Work out the finished part from the listing and answer in its coordinate system (mm). A direction names the side the tool comes from. Coordinates: 2 decimals unless noted, no trailing zeros. Loops run counter-clockwise (first coordinate to the right, second up) from the corner with the lowest first, then second, coordinate; pieces in that order, holes last. Notation, with made-up numbers: (58, -6.75) - (98, -6.75) arc R21 ccw to (98, 6.25) - close; hole circle Ø9 at (31, 38.25). An arc over 180 degrees is marked (long way). Write each question's results on one line, items separated by ' | '. Start each with the question number.
1. Determine the mould class of faces 1 (the flat face through (-5, 33.5, 6)), 2 (the flat face through (0, 32, -7.874)), 3 (the conical face through (-0.36, 33.36, 8.63)) for opening direction X: released by +X, released by -X, zero draft, split by the parting line, or undercut.
2. A cutting plane is placed at C-C on y = 29.25. Determine the outline of the cut face in (x, z).
3. Which of the six approach directions +Z, -Z, +X, -X, +Y, -Y give full straight-line access (tool end or side, diameter ignored) to faces 4 (the cylindrical face through (0, 30, -8)), 5 (the flat face through (-1, 30, -8.646)), 6 (the flat face through (7.416, 2.508, 4.325)), 7 (the flat face through (0, 3, -8.585)), 8 (the flat face through (-7.154, 3.6, 4.78))?
4. A cutting plane is placed at A-A on x = 0. Determine the outline of the cut face in (y, z).
5. A cutting plane is placed at D-D on y = 5.5. Determine the outline of the cut face in (x, z), then the cut area to 3 significant figures.
6. Each of these flat-tipped pins is pushed along its axis until it touches: P1, Ø2.5, axis at x = -0.5, y = 1.5, coming from the -Z side; P2, Ø2, axis at x = 3, z = 5, coming from the -Y side; P3, Ø1, axis at y = 4, z = 4.5, coming from the -X side; P4, Ø5, axis at y = 7, z = 6.5, coming from the +X side. Where does it stop, or does it pass through?
7. Find the intervals of material crossed by line 1 along X through (y, z) = (20.5, 0); line 2 along Y through (x, z) = (0, -8.1), in increasing order. Write a range as [from, to].
8. A cutting plane is placed at B-B on z = 0. Determine the outline of the cut face in (x, y), then the cut area to 3 significant figures.
from build123d import *

# Parameters (mm, degrees)
ESQUISSE1_R                  = 9
ESQUISSE1_R_2                = 7
BOSS_EXTRU_1_DEPTH           = 33.5
ENL_V_MAT_EXTRU_1_DEPTH      = 5
ESQUISSE3_R                  = 1
ENL_V_MAT_EXTRU_2_DEPTH      = 1.65725
ENL_V_START                  = -3
ENL_V_MAT_EXTRU_6_DEPTH      = 3
ENL_V_START_2                = -5.5
ENL_V_MAT_EXTRU_3_DEPTH      = 5.5
ENL_V_MAT_EXTRU_4_REACH      = 40.918
ENL_V_MAT_EXTRU_4_END_RADIUS = 7
ESQUISSE5_R                  = 0.75
CHANFREIN2_SIZE              = 0.5


with BuildPart() as part:
    # Esquisse1 → Boss.-Extru.1 (new body)
    with BuildSketch(Plane(origin=(0, 0, 0), x_dir=(1, 0, 0), z_dir=(0, 1, 0))):
        with Locations(Location((0, 0, 0), (0, 0, 270))):
            Circle(ESQUISSE1_R)
        with Locations(Location((0, 0, 0), (0, 0, 270))):
            Circle(ESQUISSE1_R_2, mode=Mode.SUBTRACT)
    extrude(amount=BOSS_EXTRU_1_DEPTH)

    # Esquisse2 → Enlèv. mat.-Extru.1 (cut)
    with BuildSketch(Plane.XZ):
        with BuildLine():
            Line((2.7, -8.585452813), (-2.7, -8.585452813))
            ThreePointArc((-2.7, -8.585452813), (0, -9), (2.7, -8.585452813))
        make_face()
        with BuildLine():
            Line((-8.785220239, 1.954457816), (-6.085220239, 6.630994997))
            ThreePointArc((-6.085220239, 6.630994997), (-7.794228634, 4.5), (-8.785220239, 1.954457816))
        make_face()
        with BuildLine():
            Line((6.085220239, 6.630994997), (8.785220239, 1.954457816))
            ThreePointArc((8.785220239, 1.954457816), (7.794228634, 4.5), (6.085220239, 6.630994997))
        make_face()
    extrude(amount=-ENL_V_MAT_EXTRU_1_DEPTH, mode=Mode.SUBTRACT)

    # Esquisse3 → Enlèv. mat.-Extru.2 (cut)
    with BuildSketch(Plane(origin=(-7.435220239, 0, 4.292726406), x_dir=(-0.49999999999999967, 0, -0.8660254037844389), z_dir=(0.8660254037844389, 0, -0.49999999999999967))):
        with Locations(Location((0, 2.5, 0), (0, 0, 180))):
            Circle(ESQUISSE3_R)
    extrude(amount=ENL_V_MAT_EXTRU_2_DEPTH, mode=Mode.SUBTRACT)

    # Esquisse8 → Enlèv. mat.-Extru.6 (cut)
    with BuildSketch(Plane(origin=(0, 33.5, 0), x_dir=(1, 0, 0), z_dir=(0, 1, 0)).offset(ENL_V_START)):
        with BuildLine():
            Line((-1.5, 8.874119675), (-1.5, 7.874119675))
            Line((-1.5, 7.874119675), (1.5, 7.874119675))
            Line((1.5, 7.874119675), (1.5, 8.874119675))
            ThreePointArc((1.5, 8.874119675), (0, 9), (-1.5, 8.874119675))
        make_face()
    extrude(amount=ENL_V_MAT_EXTRU_6_DEPTH, mode=Mode.SUBTRACT)

    # Esquisse4 → Enlèv. mat.-Extru.3 (cut)
    with BuildSketch(Plane(origin=(0, 33.5, 0), x_dir=(1, 0, 0), z_dir=(0, 1, 0)).offset(ENL_V_START_2)):
        with BuildLine():
            Line((2.5, 8.645808233), (-2.5, 8.645808233))
            ThreePointArc((-2.5, 8.645808233), (0, 9), (2.5, 8.645808233))
        make_face()
    extrude(amount=ENL_V_MAT_EXTRU_3_DEPTH, mode=Mode.SUBTRACT)

    # Enlèv. mat.-Extru.4: up to this cylinder (the profile starts outside it)
    enl_v_mat_extru_4_end = Plane(origin=(0, 29.25, 0), z_dir=(0, -1, 0)) * Cylinder(ENL_V_MAT_EXTRU_4_END_RADIUS, 96.836, mode=Mode.PRIVATE)
    # Esquisse5 → Enlèv. mat.-Extru.4 (cut, up to the surface)
    with BuildSketch(Plane(origin=(0, 0, -8.645808233), x_dir=(-1, 0, 0), z_dir=(0, 0, -1)), mode=Mode.PRIVATE) as enl_v_mat_extru_4_sk1:
        with Locations((0, 29.25)):
            Circle(ESQUISSE5_R)
    enl_v_mat_extru_4_tool1 = extrude(enl_v_mat_extru_4_sk1.sketch, amount=-ENL_V_MAT_EXTRU_4_REACH, mode=Mode.PRIVATE) - enl_v_mat_extru_4_end
    add(enl_v_mat_extru_4_tool1.solids().sort_by_distance((0, 29.25, -8.645808))[0], mode=Mode.SUBTRACT)

    # Chanfrein1: read off the stored shape, not the designer's step
    # Chanfrein1 outline → Chanfrein1 (revolve, cut)
    with BuildSketch(Plane.XY):
        Polygon((7, 33.5), (7, 33), (7.5, 33.5), align=None)
        Polygon((9.000000072, 33.5), (8.5, 33.5), (9, 33), align=None)
        Polygon((9.000000072, 0), (9.000000072, 0.500000072), (8.5, 0), align=None)
    revolve(axis=Axis((0, 0, 0), (0, 1, 0)), mode=Mode.SUBTRACT)

    # Chanfrein2
    chanfrein2_edges = [part.edges().sort_by_distance(p)[0] for p in [
        (0, 0, -7),
    ]]
    chamfer(chanfrein2_edges, length=CHANFREIN2_SIZE)


solid = part.part
Values:
1) face 1: zero draft | face 2: undercut | face 3: split by the parting line
2) outline: (-2.5, -8.65) - (-0.75, -8.65) - (-0.75, -6.96) arc R7 cw (long way) to (0.75, -6.96) - (0.75, -8.65) - (2.5, -8.65) arc R9 ccw (long way) to start
3) face 4: -Z | face 5: -Z, +X, -X, +Y | face 6: +Z, +X, -Y | face 7: -Z, +X, -X, -Y | face 8: +Z, -X, -Y
4) outline: (0, -8.5) - (0.09, -8.59) - (5, -8.59) - (5, -9) - (28, -9) - (28, -8.65) - (28.5, -8.65) - (28.5, -7) - (0.5, -7) - (0, -7.5) - close; (0, 7.5) - (0.5, 7) - (33, 7) - (33.5, 7.5) - (33.5, 8.5) - (33, 9) - (0.5, 9) - (0, 8.5) - close; (30, -8.65) - (30.5, -8.65) - (30.5, -7.87) - (33.5, -7.87) - (33.5, -7.5) - (33, -7) - (30, -7) - close
5) outline: circle Ø18 at (0, 0); hole circle Ø14 at (0, 0) | area: 101 mm^2
6) P1: z = -8.59 | P2: through | P3: x = -7.6 | P4: x = 8.06
7) line 1: [-9, -7], [7, 9] | line 2: [0, 28.5], [30, 30.5]
8) outline: (-9, 0.5) - (-8.5, 0) - (-7.5, 0) - (-7, 0.5) - (-7, 33) - (-7.5, 33.5) - (-8.5, 33.5) - (-9, 33) - close; (7, 0.5) - (7.5, 0) - (8.5, 0) - (9, 0.5) - (9, 33) - (8.5, 33.5) - (7.5, 33.5) - (7, 33) - close | area: 133 mm^2
